from build123d import *

# Parameters (mm, degrees)
SKETCH1_W           = 20
SKETCH1_H           = 40
BOSS_EXTRUDE1_DEPTH = 5
FILLET2_R           = 10
SKETCH2_R           = 2.5
CUT_EXTRUDE1_DEPTH  = 23.912878475
SKETCH3_R           = 2.55
CUT_EXTRUDE2_DEPTH  = 5


with BuildPart() as part:
    # Sketch1 → Boss-Extrude1 (new body)
    with BuildSketch(Plane.XY):
        Rectangle(SKETCH1_W, SKETCH1_H)
    extrude(amount=BOSS_EXTRUDE1_DEPTH)

    # Fillet2
    fillet2_edges = [part.edges().sort_by_distance(p)[0] for p in [
        (-10, 20, 2.5),
        (10, 20, 2.5),
    ]]
    fillet(fillet2_edges, radius=FILLET2_R - 0.0001)  # a hair under: the kernel refuses the full size

    # Sketch2 → Cut-Extrude1 (cut, through all)
    with BuildSketch(Plane(origin=(0, 0, 0), x_dir=(-1, 0, 0), z_dir=(0, 0, -1))):
        with Locations((0, 10)):
            Circle(SKETCH2_R)
    extrude(amount=-CUT_EXTRUDE1_DEPTH, mode=Mode.SUBTRACT)

    # Sketch3 → Cut-Extrude2 (cut)
    with BuildSketch(Plane(origin=(0, 0, 0), x_dir=(-1, 0, 0), z_dir=(0, 0, -1))):
        with Locations((-5, -10)):
            Circle(SKETCH3_R)
        with Locations((5, -10)):
            Circle(SKETCH3_R)
    extrude(amount=-CUT_EXTRUDE2_DEPTH, mode=Mode.SUBTRACT)


solid = part.part
For this review, take the finished solid that the model builds, in its own axes (mm). Round coordinates to 2 decimals unless told otherwise and drop trailing zeros. Loops run counter-clockwise (first coordinate to the right, second up) from the corner with the lowest first, then second, coordinate; pieces in that order, holes last. Notation, with made-up numbers: (47.5, 40) - (79.5, 40) arc R14 ccw to (79.5, 67) - close; hole circle Ø7 at (40.5, 85). An arc over 180 degrees is marked (long way). One line per item, written item: value. Start each with the question number.
Item 1: Clearance check with a flat-ended pin moving along its axis: pin 1 Ø4.5 at (x, y) = (0, 10) entering from +Z. State where the tip first meets the part, or that it passes through.
Item 2: Take a section at D-D (x = -7). Give the boundary of the cut face in (y, z), plus the area to 3 significant figures.
Item 3: For L1, parallel to Y at x = 0, z = 2.55; L2, parallel to Y at x = 1, z = 2.9; L3, parallel to X at y = 8.5, z = 1.85, list the stretches that pass through material, from the lowest coordinate up.
Item 4: Take a section at B-B (y = 8). Give the boundary of the cut face in (x, z).
Item 5: Take a section at C-C (z = 3.2). State how many separate pieces and enclosed holes the cut face has, plus the area to 3 significant figures.
Item 6: Take a section at A-A (y = -10). Give the boundary of the cut face in (x, z).
Item 7: The part is to be moulded in two halves that separate along X. For faces 1 (the cylindrical face through (-6.18, -12.26, 2.46)), 2 (the cylindrical face through (-7.15, 16.99, 2.54)), 3 (the flat face through (0, -20, 2)), 4 (the cylindrical face through (3.82, -12.26, 2.46)), say which applies: +X half, -X half, draft (parallel to the pull), parting line (faces both ways), or undercut.
Answer below:
1. pin 1: passes through
2. outline: (-20, 0) - (-11.58, 0) - (-11.58, 5) - (-20, 5) - close; (-8.42, 0) - (17.14, 0) - (17.14, 5) - (-8.42, 5) - close
2. area: 170 mm2
3. L1: y = -20 to 7.5, 12.5 to 20
3. L2: y = -20 to 7.71, 12.29 to 19.95
3. L3: x = -10 to -2, 2 to 10
4. outline: (-10, 0) - (-1.5, 0) - (-1.5, 5) - (-10, 5) - close; (1.5, 0) - (10, 0) - (10, 5) - (1.5, 5) - close
5. separate pieces: 1
5. enclosed holes: 3
5. area: 697 mm2
6. outline: (-10, 0) - (-7.55, 0) - (-7.55, 5) - (-10, 5) - close; (-2.45, 0) - (2.45, 0) - (2.45, 5) - (-2.45, 5) - close; (7.55, 0) - (10, 0) - (10, 5) - (7.55, 5) - close
7. face 1: undercut
7. face 2: -X half
7. face 3: draft
7. face 4: undercut
